Autodesk Inventor part; units mm, degrees
ref_plane "YZ Plane" through (0, 0, 0) normal (1, 0, 0) x (0, 1, 0)
ref_plane "XZ Plane" through (0, 0, 0) normal (0, 1, 0) x (-1, 0, 0)
ref_plane "XY Plane" through (0, 0, 0) normal (0, 0, 1) x (1, 0, 0)
sketch "Sketch1" plane through (0, 0, 0) normal (0, 1, 0) x (-1, 0, 0)
  line L0 (0, 0) -> (-10, 0)
  line L1 (-10, 0) -> (-10, -50)
  line L2 (-10, -50) -> (0, -50)
  line L3 (0, -50) -> (0, 0)
  dimension "d0" = 10
  dimension "d1" = 50
extrude "Extrusion1" add sketch "Sketch1" along normal blind 3
sketch "Sketch2" plane through (0, 3, 0) normal (0, 1, 0) x (1, 0, 0)
  line L0 (0, 0) -> (10, 0)
  line L1 (10, 0) -> (10, 50)
  line L2 (0, 0) -> (10, 0)
  line L3 (10, 0) -> (10, 5)
  line L4 (10, 5) -> (0, 5)
  line L5 (0, 5) -> (0, 0)
  line L6 (0, 50) -> (0, 0)
  line L7 (0, 50) -> (10, 50)
  line L8 (10, 50) -> (10, 45)
  line L9 (10, 45) -> (0, 45)
  line L10 (0, 45) -> (0, 50)
  dimension "d4" = 5
  dimension "d5" = 5
extrude "Extrusion2" add sketch "Sketch2" along normal blind 12 contours L5 L4 L1 L0 | L6 L7 L1 L9
equation "\"BendRadius\" = Thickness"
equation "\"BendReliefWidth\" = Thickness"
equation "\"BendReliefDepth\" = 0.5 * Thickness"
equation "\"CornerReliefSize\" = 4 * Thickness"
equation "\"MinimumRemnant\" = 2 * Thickness"
equation "\"TransitionRadius\" = BendRadius"
equation "\"JacobiRadiusSize\" = BendRadius"
equation "\"GapSize\" = Thickness"
Work out the finished part from the listing and answer in its coordinate system (mm). A direction names the side the tool comes from. Coordinates: 2 decimals unless noted, no trailing zeros. Loops run counter-clockwise (first coordinate to the right, second up) from the corner with the lowest first, then second, coordinate; pieces in that order, holes last. Notation, with made-up numbers: M -20,63.5 L -7,63.5 A21 ccw -7,93.5 Z; hole C 32,83 d3. An arc over 180 degrees is marked long. Use CSV: the item, a comma, the result in double quotes. Start each with the question number.
(1) Given pin 1 Ø3 at (x, z) = (6, -25.5) entering from +Y; pin 2 Ø1 at (x, y) = (5.5, 6) entering from +Z, each flat-ended and moving along its own axis, determine where each tip first touches the part or whether it passes through.
(2) Consider line 1 (Z direction, x = 8.5, y = 8); line 2 (Y direction, x = 4.5, z = -10.5). Determine where each line is inside the solid, lowest interval first.
(3) Find section A-A, the plane y = 5.75. Give the vertices of the cut face in (x, z), then the cut area to 3 significant figures.
(4) Find section C-C, the plane z = -43.5. Give the vertices of the cut face in (x, y).
(5) For faces 1 (the face through (5, 7, 0)), 2 (the face through (5, 9, -45)), determine the directions among +Z, -Z, +X, -X, +Y, -Y from which every point of the face is accessible in a straight line to the end or side of a thin tool.
(6) Find section B-B, the plane x = 8.25. Give the vertices of the cut face in (y, z), then the cut area to 3 significant figures.
(7) For a pull along Z with two mould halves and no side action, classify faces 3 (the face through (10, 2, -25)), 4 (the face through (5, 7, -50)), 5 (the face through (5, 9, -5)) as +Z half, -Z half, draft (parallel to the pull), parting line (faces both ways), or undercut.
Recorded:
1,pin 1,"stops at y = 3"
1,pin 2,"stops at z = 0"
2,line 1,"z = -50 to -45, -5 to 0"
2,line 2,"y = 0 to 3"
3,outline,"M 0,-50 L 10,-50 L 10,-45 L 0,-45 Z; M 0,-5 L 10,-5 L 10,0 L 0,0 Z"
3,area,"100 mm^2"
4,outline,"M 0,0 L 10,0 L 10,3 L 0,3 Z"
5,face 1,"+Z, +X, -X, +Y, -Y"
5,face 2,"+X, -X, +Y"
6,outline,"M 0,-50 L 15,-50 L 15,-45 L 3,-45 L 3,-5 L 15,-5 L 15,0 L 0,0 Z"
6,area,"270 mm^2"
7,face 3,"draft"
7,face 4,"-Z half"
7,face 5,"undercut"
